Input: part model. Units: mm. Frame: model coordinates. Give positions to 0.01 mm unless a question says otherwise; leave off trailing zeros. Order: outer loops, then holes, each group sorted by start corner. A loop starts at its lowest first (then second) coordinate and runs counter-clockwise, first axis right, second up. Notation, with made-up numbers: M -5.5,-36.5 L 48.5,-36.5 A5 ccw 48.5,-30.5 Z; hole C -35.75,6.5 d7. An arc over 180 degrees is marked long. Use a Markdown table: item, result.
from build123d import *

# Parameters (mm, degrees)
PAD_DEPTH    = 35
SKETCH001_R  = 3
POCKET_DEPTH = 10
FILLET_R     = 5


with BuildPart() as part:
    # Sketch → Pad (new body)
    with BuildSketch(Plane.XY):
        with BuildLine():
            Line((-31.743039, 5.632756), (28.256961, 5.632756))
            Line((28.256961, 5.632756), (28.256961, -4.367244))
            Line((2.256961, -4.367244), (28.256961, -4.367244))
            ThreePointArc((2.256961, -4.367244), (-1.743039, -0.367244), (-5.743039, -4.367244))
            Line((-31.743039, -4.367244), (-5.743039, -4.367244))
            Line((-31.743039, -4.367244), (-31.743039, 5.632756))
        make_face()
    extrude(amount=PAD_DEPTH)

    # Sketch001 → Pocket (cut)
    with BuildSketch(Plane(origin=(0, 5.632756, 0), x_dir=(-1, 0, 0), z_dir=(0, 1, 0))):
        with Locations((-16.256961, 23)):
            Circle(SKETCH001_R)
        with Locations((19.743039, 23)):
            Circle(SKETCH001_R)
    extrude(amount=-POCKET_DEPTH, mode=Mode.SUBTRACT)

    # Fillet
    fillet_edges = [part.edges().sort_by_distance(p)[0] for p in [
        (-1.743039, 5.632756, 35),
    ]]
    fillet(fillet_edges, radius=FILLET_R)


solid = part.part
1) Material intervals for line 1 (X direction, y = 1, z = 24.5); line 2 (X direction, y = -2.75, z = 33); line 3 (X direction, y = -1.5, z = 5), sorted ascending. Write a range as from..to.
Response values:
| item | result |
|---|---|
| line 1 | x = -31.74..-22.34, -17.14..13.66, 18.86..28.26 |
| line 2 | x = -31.74..-5.4, 1.92..28.26 |
| line 3 | x = -31.74..-4.53, 1.05..28.26 |
2) Cut plane D-D on z = 5.5. Return loops of the section in (x, y), and give its area (3 significant figures).
Response values:
| item | result |
|---|---|
| outline | M -31.74,-4.37 L -5.74,-4.37 A4 cw 2.26,-4.37 L 28.26,-4.37 L 28.26,5.63 L -31.74,5.63 Z |
| area | 575 mm² |
3) Cut plane C-C on y = 2.75. Return loops of the section in (x, z).
Response values:
| item | result |
|---|---|
| outline | M -31.74,0 L 28.26,0 L 28.26,34.53 L -31.74,34.53 Z; hole C -19.74,23 d6; hole C 16.26,23 d6 |
4) Cut plane B-B on y = -3. Return loops of the section in (x, z), and give its area (3 significant figures).
Response values:
| item | result |
|---|---|
| outline | M -31.74,0 L -5.5,0 L -5.5,35 L -31.74,35 Z; M 2.02,0 L 28.26,0 L 28.26,35 L 2.02,35 Z; hole C -19.74,23 d6; hole C 16.26,23 d6 |
| area | 1,780 mm² |
5) Cut plane A-A on z = 23. Return loops of the section in (x, y), and give its area (3 significant figures).
Response values:
| item | result |
|---|---|
| outline | M -31.74,-4.37 L -22.74,-4.37 L -22.74,5.63 L -31.74,5.63 Z; M -16.74,-4.37 L -5.74,-4.37 A4 cw 2.26,-4.37 L 13.26,-4.37 L 13.26,5.63 L -16.74,5.63 Z; M 19.26,-4.37 L 28.26,-4.37 L 28.26,5.63 L 19.26,5.63 Z |
| area | 455 mm² |
6) First-contact query: pin 1 Ø8 at (x, z) = (-19.74, 23) entering from +Y. Flat tip, straight axial feed; report the tip coordinate or a pass-through.
Response values:
| item | result |
|---|---|
| pin 1 | stops at y = 5.63 |
7) Mould query, pull axis X, two halves, no side actions, for faces 1 (the face through (-16.746, 0.703, 23.132)), 2 (the face through (28.257, 1, 17)), 3 (the face through (15, -4.367, 17)). Classes: released by +X, released by -X, zero draft, split by the parting line, or undercut.
Response values:
| item | result |
|---|---|
| face 1 | undercut |
| face 2 | released by +X |
| face 3 | zero draft |
